Verification items for the finished model (mm, model axes). Round coordinates to 2 decimals unless told otherwise and drop trailing zeros. Write each loop counter-clockwise with the first axis right and the second up, starting at its lowest first coordinate (ties: lowest second). Pieces come first, ordered by that corner, then holes. Notation, with made-up numbers: M 10.5,-39.5 L 39.5,-39.5 A22 ccw 39.5,-3.5 Z; hole C 27.25,47.5 d7. An arc over 180 degrees is marked long. Use a Markdown table: item, result. Add a question column.
from build123d import *

# Parameters (mm, degrees)
SKETCH1_R                       = 40
SKETCH1_R_2                     = 10
BOSS_EXTRUDE1_DEPTH             = 4
M4X0_7_TAPPED_HOLE2_D           = 3.3
M4X0_7_TAPPED_HOLE2_CSINK_D     = 4.05
M4X0_7_TAPPED_HOLE2_CSINK_ANGLE = 90
M4X0_7_TAPPED_HOLE3_D           = 3.3
M4X0_7_TAPPED_HOLE3_CSINK_D     = 4.05
M4X0_7_TAPPED_HOLE3_CSINK_ANGLE = 90
CIRPATTERN1_COUNT               = 12
FILLET1_R                       = 2


with BuildPart() as part:
    # Sketch1 → Boss-Extrude1 (new, symmetric)
    with BuildSketch(Plane.XY):
        Circle(SKETCH1_R)
        Circle(SKETCH1_R_2, mode=Mode.SUBTRACT)
        with BuildLine():
            Line((-2.5, 28.641098093), (-2.5, 16.30950643))
            ThreePointArc((-2.5, 16.30950643), (-4.270514244, 15.937776134), (-5.989689706, 15.374446892))
            Line((-5.989689706, 15.374446892), (-12.155485537, 26.053918541))
            ThreePointArc((-12.155485537, 26.053918541), (-7.441047547, 27.770367506), (-2.5, 28.641098093))
        make_face(mode=Mode.SUBTRACT)
        with BuildLine():
            Line((2.5, 28.641098093), (2.5, 16.30950643))
            ThreePointArc((2.5, 16.30950643), (4.270514244, 15.937776134), (5.989689706, 15.374446892))
            Line((5.989689706, 15.374446892), (12.155485537, 26.053918541))
            ThreePointArc((12.155485537, 26.053918541), (7.441047547, 27.770367506), (2.5, 28.641098093))
        make_face(mode=Mode.SUBTRACT)
        with BuildLine():
            Line((16.485612556, 23.553918541), (10.319816725, 12.874446892))
            ThreePointArc((10.319816725, 12.874446892), (11.66726189, 11.66726189), (12.874446892, 10.319816725))
            Line((12.874446892, 10.319816725), (23.553918541, 16.485612556))
            ThreePointArc((23.553918541, 16.485612556), (20.329319959, 20.329319959), (16.485612556, 23.553918541))
        make_face(mode=Mode.SUBTRACT)
        with BuildLine():
            Line((26.053918541, 12.155485537), (15.374446892, 5.989689706))
            ThreePointArc((15.374446892, 5.989689706), (15.937776134, 4.270514244), (16.30950643, 2.5))
            Line((16.30950643, 2.5), (28.641098093, 2.5))
            ThreePointArc((28.641098093, 2.5), (27.770367506, 7.441047547), (26.053918541, 12.155485537))
        make_face(mode=Mode.SUBTRACT)
        with BuildLine():
            Line((28.641098093, -2.5), (16.30950643, -2.5))
            ThreePointArc((16.30950643, -2.5), (15.937776134, -4.270514244), (15.374446892, -5.989689706))
            Line((15.374446892, -5.989689706), (26.053918541, -12.155485537))
            ThreePointArc((26.053918541, -12.155485537), (27.770367506, -7.441047547), (28.641098093, -2.5))
        make_face(mode=Mode.SUBTRACT)
        with BuildLine():
            Line((23.553918541, -16.485612556), (12.874446892, -10.319816725))
            ThreePointArc((12.874446892, -10.319816725), (11.66726189, -11.66726189), (10.319816725, -12.874446892))
            Line((10.319816725, -12.874446892), (16.485612556, -23.553918541))
            ThreePointArc((16.485612556, -23.553918541), (20.329319959, -20.329319959), (23.553918541, -16.485612556))
        make_face(mode=Mode.SUBTRACT)
        with BuildLine():
            Line((12.155485537, -26.053918541), (5.989689706, -15.374446892))
            ThreePointArc((5.989689706, -15.374446892), (4.270514244, -15.937776134), (2.5, -16.30950643))
            Line((2.5, -16.30950643), (2.5, -28.641098093))
            ThreePointArc((2.5, -28.641098093), (7.441047547, -27.770367506), (12.155485537, -26.053918541))
        make_face(mode=Mode.SUBTRACT)
        with BuildLine():
            Line((-2.5, -28.641098093), (-2.5, -16.30950643))
            ThreePointArc((-2.5, -16.30950643), (-4.270514244, -15.937776134), (-5.989689706, -15.374446892))
            Line((-5.989689706, -15.374446892), (-12.155485537, -26.053918541))
            ThreePointArc((-12.155485537, -26.053918541), (-7.441047547, -27.770367506), (-2.5, -28.641098093))
        make_face(mode=Mode.SUBTRACT)
        with BuildLine():
            Line((-16.485612556, -23.553918541), (-10.319816725, -12.874446892))
            ThreePointArc((-10.319816725, -12.874446892), (-11.66726189, -11.66726189), (-12.874446892, -10.319816725))
            Line((-12.874446892, -10.319816725), (-23.553918541, -16.485612556))
            ThreePointArc((-23.553918541, -16.485612556), (-20.329319959, -20.329319959), (-16.485612556, -23.553918541))
        make_face(mode=Mode.SUBTRACT)
        with BuildLine():
            Line((-26.053918541, -12.155485537), (-15.374446892, -5.989689706))
            ThreePointArc((-15.374446892, -5.989689706), (-15.937776134, -4.270514244), (-16.30950643, -2.5))
            Line((-16.30950643, -2.5), (-28.641098093, -2.5))
            ThreePointArc((-28.641098093, -2.5), (-27.770367506, -7.441047547), (-26.053918541, -12.155485537))
        make_face(mode=Mode.SUBTRACT)
        with BuildLine():
            Line((-28.641098093, 2.5), (-16.30950643, 2.5))
            ThreePointArc((-16.30950643, 2.5), (-15.937776134, 4.270514244), (-15.374446892, 5.989689706))
            Line((-15.374446892, 5.989689706), (-26.053918541, 12.155485537))
            ThreePointArc((-26.053918541, 12.155485537), (-27.770367506, 7.441047547), (-28.641098093, 2.5))
        make_face(mode=Mode.SUBTRACT)
        with BuildLine():
            Line((-23.553918541, 16.485612556), (-12.874446892, 10.319816725))
            ThreePointArc((-12.874446892, 10.319816725), (-11.66726189, 11.66726189), (-10.319816725, 12.874446892))
            Line((-10.319816725, 12.874446892), (-16.485612556, 23.553918541))
            ThreePointArc((-16.485612556, 23.553918541), (-20.329319959, 20.329319959), (-23.553918541, 16.485612556))
        make_face(mode=Mode.SUBTRACT)
    extrude(amount=BOSS_EXTRUDE1_DEPTH, both=True)

    # M4x0.7 Tapped Hole2 (through all)
    with Locations(Plane.XY.offset(4)):
        with Locations((-8.838834765, 8.838834765), (-8.838834765, -8.838834765), (8.838834765, -8.838834765), (8.838834765, 8.838834765)):
            CounterSinkHole(M4X0_7_TAPPED_HOLE2_D / 2, M4X0_7_TAPPED_HOLE2_CSINK_D / 2, counter_sink_angle=M4X0_7_TAPPED_HOLE2_CSINK_ANGLE)

    # M4x0.7 Tapped Hole3 (through all)
    with Locations(Plane.XY.offset(4)):
        with Locations((0, 36.25)):
            m4x0_7_tapped_hole3 = CounterSinkHole(M4X0_7_TAPPED_HOLE3_D / 2, M4X0_7_TAPPED_HOLE3_CSINK_D / 2, counter_sink_angle=M4X0_7_TAPPED_HOLE3_CSINK_ANGLE)

    # CirPattern1: M4x0.7 Tapped Hole3 ×12 about axis
    cirpattern1_axis = Axis((0, 0, 0), (0, 0, 1))
    for i in range(1, CIRPATTERN1_COUNT):
        add(m4x0_7_tapped_hole3.rotate(cirpattern1_axis, i * 360 / CIRPATTERN1_COUNT), mode=Mode.SUBTRACT)

    # Fillet1
    fillet1_edges = [part.edges().sort_by_distance(p)[0] for p in [
        (28.641098093, 2.5, 0),
        (26.053918541, 12.155485537, 0),
        (15.374446892, 5.989689706, 0),
        (16.30950643, 2.5, 0),
        (16.485612556, -23.553918541, 0),
        (23.553918541, -16.485612556, 0),
        (12.874446892, -10.319816725, 0),
        (10.319816725, -12.874446892, 0),
        (-26.053918541, 12.155485537, 0),
        (-28.641098093, 2.5, 0),
        (-16.30950643, 2.5, 0),
        (2.5, -28.641098093, 0),
        (12.155485537, -26.053918541, 0),
        (5.989689706, -15.374446892, 0),
        (2.5, -16.30950643, 0),
        (-15.374446892, 5.989689706, 0),
        (-23.553918541, -16.485612556, 0),
        (-16.485612556, -23.553918541, 0),
        (-10.319816725, -12.874446892, 0),
        (-12.874446892, -10.319816725, 0),
        (-28.641098093, -2.5, 0),
        (-26.053918541, -12.155485537, 0),
        (-15.374446892, -5.989689706, 0),
        (-16.30950643, -2.5, 0),
        (26.053918541, -12.155485537, 0),
        (28.641098093, -2.5, 0),
        (16.30950643, -2.5, 0),
        (15.374446892, -5.989689706, 0),
        (12.155485537, 26.053918541, 0),
        (2.5, 28.641098093, 0),
        (2.5, 16.30950643, 0),
        (5.989689706, 15.374446892, 0),
        (-12.155485537, -26.053918541, 0),
        (-2.5, -28.641098093, 0),
        (-2.5, -16.30950643, 0),
        (-5.989689706, -15.374446892, 0),
        (-5.989689706, 15.374446892, 0),
        (-2.5, 16.30950643, 0),
        (-2.5, 28.641098093, 0),
        (-12.155485537, 26.053918541, 0),
        (-16.485612556, 23.553918541, 0),
        (-23.553918541, 16.485612556, 0),
        (-12.874446892, 10.319816725, 0),
        (-10.319816725, 12.874446892, 0),
        (23.553918541, 16.485612556, 0),
        (16.485612556, 23.553918541, 0),
        (10.319816725, 12.874446892, 0),
        (12.874446892, 10.319816725, 0),
    ]]
    fillet(fillet1_edges, radius=FILLET1_R)


solid = part.part
1. Cross-section at A-A on y = 0. Enter the section's corners in (x, z) (3 decimals), plus the area to 3 significant figures.
2. Cross-section at C-C on y = -36.25. Enter the section's corners in (x, z) (3 decimals).
3. Scan lines: line 1 along Y through (x, z) = (0, -1.5); line 2 along X through (y, z) = (-7.5, 1.75); line 3 along Y through (x, z) = (-8, -1.5). Record each from-to range of solid material in increasing order. Write a range as from..to.
4. Depth check by flat-ended pin: pin 1 Ø1 at (x, z) = (30.5, -2.5) entering from -Y; pin 2 Ø2.5 at (x, y) = (31.39, 18.13) entering from -Z; pin 3 Ø1 at (x, z) = (5.5, 0) entering from -Y; pin 4 Ø4 at (y, z) = (-20.5, 0.5) entering from +X. Enter the tip coordinate at first touch or a pass-through.
Answer:
| question | item | result |
|---|---|---|
| 1 | outline | M -40,-4 L -37.9,-4 L -37.9,3.625 L -38.275,4 L -40,4 Z; M -34.6,-4 L -10,-4 L -10,4 L -34.225,4 L -34.6,3.625 Z; M 10,-4 L 34.6,-4 L 34.6,3.625 L 34.225,4 L 10,4 Z; M 37.9,-4 L 40,-4 L 40,4 L 38.275,4 L 37.9,3.625 Z |
| 1 | area | 427 mm^2 |
| 2 | outline | M -16.91,-4 L -1.65,-4 L -1.65,3.625 L -2.025,4 L -16.91,4 Z; M 1.65,-4 L 16.91,-4 L 16.91,4 L 2.025,4 L 1.65,3.625 Z |
| 3 | line 1 | y = -40..-37.9, -34.6..-10, 10..34.6, 37.9..40 |
| 3 | line 2 | x = -39.29..-27.75, -17.99..-9.8, -7.87..-6.61, 6.61..7.87, 9.8..17.99, 27.75..39.29 |
| 3 | line 3 | y = -39.19..-27.61, -18.86..-10.26, -7.42..-6, 6..7.42, 10.26..18.86, 27.61..39.19 |
| 4 | pin 1 | stops at y = -26.46 |
| 4 | pin 2 | passes through |
| 4 | pin 3 | stops at y = -39.69 |
| 4 | pin 4 | stops at x = 35.46 |
